Check sheet for the modelled part. Datum: model origin and axes. Units: mm. Face numbers are marked on the shaded views. Round coordinates to 2 decimals unless told otherwise and drop trailing zeros. Write each loop counter-clockwise with the first axis right and the second up, starting at its lowest first coordinate (ties: lowest second). Pieces come first, ordered by that corner, then holes. Notation, with made-up numbers: (-31.75, 80) -> (-19.75, 80) arc R22 cw to (-19.75, 107) -> close; hole circle Ø3 at (-9.5, 43.5). An arc over 180 degrees is marked (long way). One line per item, written item: value.
from build123d import *

# Parameters (mm, degrees)
F1_DEPTH  = 1600
F3_DEPTH  = 1.5
F5_DEPTH  = 13.5
F6_W      = 507
F6_H      = 1.5
F7_ANGLE  = 90
F8_W      = 507
F8_H      = 1.5
F9_DEPTH  = 13.5
F10_W     = 1.5
F10_H     = 28.5
F12_W     = 1.5
F12_H     = 28.5
F15_DEPTH = 1.5
F16_W     = 500
F16_H     = 1.5
F17_DEPTH = 38.5
F18_R     = 5
F19_W     = 30
F19_H     = 30
F20_DEPTH = 865.5
F21_W     = 490
F21_H     = 30
F22_DEPTH = 936.5
F23_W     = 430
F23_H     = 30
F24_DEPTH = 30


with BuildPart() as f1:
    # F0 (on Front) → F1 (new body)
    with BuildSketch(Plane.XZ):
        with BuildLine():
            Line((-285, 28.5), (-285, 0))
            Line((-285, 0), (-283.5, 0))
            Line((-283.5, 0), (-283.5, 28.5))
            Line((-283.5, 28.5), (-256.5, 28.5))
            Line((-256.5, 28.5), (-256.5, 3))
            ThreePointArc((-256.5, 3), (-255.6213203436, 0.8786796564), (-253.5, 0))
            Line((-253.5, 0), (253.5, 0))
            ThreePointArc((253.5, 0), (255.6213203436, 0.8786796564), (256.5, 3))
            Line((256.5, 3), (256.5, 28.5))
            Line((256.5, 28.5), (283.5, 28.5))
            Line((283.5, 28.5), (283.5, 0))
            Line((283.5, 0), (285, 0))
            Line((285, 0), (285, 28.5))
            ThreePointArc((285, 28.5), (284.5606601718, 29.5606601718), (283.5, 30))
            Line((283.5, 30), (256.5, 30))
            ThreePointArc((256.5, 30), (255.4393398282, 29.5606601718), (255, 28.5))
            Line((255, 28.5), (255, 3))
            ThreePointArc((255, 3), (254.5606601718, 1.9393398282), (253.5, 1.5))
            Line((253.5, 1.5), (-253.5, 1.5))
            ThreePointArc((-253.5, 1.5), (-254.5606601718, 1.9393398282), (-255, 3))
            Line((-255, 3), (-255, 28.5))
            ThreePointArc((-255, 28.5), (-255.4393398282, 29.5606601718), (-256.5, 30))
            Line((-256.5, 30), (-283.5, 30))
            ThreePointArc((-283.5, 30), (-284.5606601718, 29.5606601718), (-285, 28.5))
        make_face()
    extrude(amount=F1_DEPTH)

    # F2 (on face) → F3 (join)
    with BuildSketch(Plane(origin=(0, 0, 0), x_dir=(-1, 0, 0), z_dir=(0, 1, 0))):
        with BuildLine():
            ThreePointArc((-283.5, 30), (-284.5606601718, 29.5606601718), (-285, 28.5))
            Line((-285, 28.5), (-285, 0))
            Line((-285, 0), (285, 0))
            Line((285, 0), (285, 28.5))
            ThreePointArc((285, 28.5), (284.5606601718, 29.5606601718), (283.5, 30))
            Line((283.5, 30), (-283.5, 30))
        make_face()
    extrude(amount=F3_DEPTH)

    # F4 (on face) → F5 (join)
    with BuildSketch(Plane.XZ.offset(1600)):
        with BuildLine():
            ThreePointArc((253.5, 0), (255.6213203436, 0.8786796564), (256.5, 3))
            Line((256.5, 3), (256.5, 15))
            Line((256.5, 15), (255, 15))
            Line((255, 15), (255, 3))
            ThreePointArc((255, 3), (254.5606601718, 1.9393398282), (253.5, 1.5))
            Line((253.5, 1.5), (-253.5, 1.5))
            ThreePointArc((-253.5, 1.5), (-254.5606601718, 1.9393398282), (-255, 3))
            Line((-255, 3), (-255, 15))
            Line((-255, 15), (-256.5, 15))
            Line((-256.5, 15), (-256.5, 3))
            ThreePointArc((-256.5, 3), (-255.6213203436, 0.8786796564), (-253.5, 0))
            Line((-253.5, 0), (253.5, 0))
        make_face()
    extrude(amount=F5_DEPTH)

    # F6 (on face) → F7 (revolve)
    with BuildSketch(Plane.XZ.offset(1613.5)):
        with Locations((0, 0.75)):
            Rectangle(F6_W, F6_H)
    revolve(axis=Axis((0, -1613.5, 0), (1, 0, 0)), revolution_arc=F7_ANGLE)

    # F8 (on face) → F9 (join)
    with BuildSketch(Plane(origin=(0, 0, 0), x_dir=(1, 0, 0), z_dir=(0, 0, -1))):
        with Locations((0, 1614.25)):
            Rectangle(F8_W, F8_H)
    extrude(amount=F9_DEPTH)

    # F10 (on face) → F11 (join, up to the next surface of F1)
    with BuildSketch(Plane(origin=(283.5, 0, 0), x_dir=(0, -1, 0), z_dir=(-1, 0, 0))):
        with Locations((1599.25, 14.25)):
            Rectangle(F10_W, F10_H)
    extrude(until=Until.NEXT)

    # F12 (on face) → F13 (join, up to the next surface of F1)
    with BuildSketch(Plane.YZ.offset(-283.5)):
        with Locations((-1599.25, 14.25)):
            Rectangle(F12_W, F12_H)
    extrude(until=Until.NEXT)

    # F14 (on face) → F15 (join)
    with BuildSketch(Plane(origin=(0, 0, 0), x_dir=(1, 0, 0), z_dir=(0, 0, -1))):
        with BuildLine():
            Line((250, 1570.5), (250, 1605.5))
            Line((250, 1605.5), (-250, 1605.5))
            Line((-250, 1605.5), (-250, 1570.5))
            ThreePointArc((-250, 1570.5), (-248.5355339059, 1566.9644660941), (-245, 1565.5))
            Line((-245, 1565.5), (245, 1565.5))
            ThreePointArc((245, 1565.5), (248.5355339059, 1566.9644660941), (250, 1570.5))
        make_face()
    extrude(amount=F15_DEPTH)

    # F16 (on face) → F17 (join)
    with BuildSketch(Plane(origin=(0, 0, -1.5), x_dir=(1, 0, 0), z_dir=(0, 0, -1))):
        with Locations((0, 1604.75)):
            Rectangle(F16_W, F16_H)
    extrude(amount=F17_DEPTH)

    # F18
    f18_edges = [f1.edges().sort_by_distance(p)[0] for p in [
        (-250, -1604.75, -40),
        (250, -1604.75, -40),
    ]]
    fillet(f18_edges, radius=F18_R)

    # F19 (on face) → F20 (join)
    with BuildSketch(Plane(origin=(0, 0, 0), x_dir=(1, 0, 0), z_dir=(0, 0, -1))):
        with Locations((-230, 1525)):
            Rectangle(F19_W, F19_H)
        with Locations((230, 1525)):
            Rectangle(F19_W, F19_H)
    extrude(amount=F20_DEPTH)

    # F21 (on face) → F22 (join)
    with BuildSketch(Plane.XZ.offset(1540)):
        with Locations((0, -730.5)):
            Rectangle(F21_W, F21_H)
    extrude(amount=-F22_DEPTH)

    # F23 (on face) → F24 (join)
    with BuildSketch(Plane(origin=(0, -603.5, 0), x_dir=(-1, 0, 0), z_dir=(0, 1, 0))):
        with Locations((0, -730.5)):
            Rectangle(F23_W, F23_H)
    extrude(amount=F24_DEPTH)


solid = f1.part
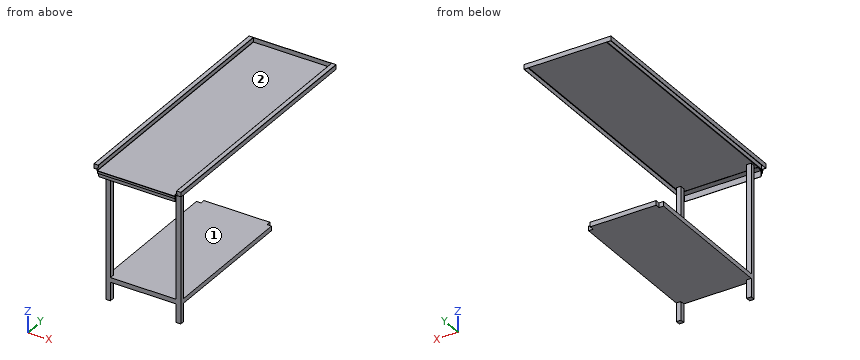
Item 1: Sectioned sample at A-A (y = -1485). Enter the section's corners in (x, z), then the cut area to 3 significant figures.
Result set:
outline: (-285, 0) -> (-283.5, 0) -> (-283.5, 28.5) -> (-256.5, 28.5) -> (-256.5, 3) arc R3 ccw to (-253.5, 0) -> (253.5, 0) arc R3 ccw to (256.5, 3) -> (256.5, 28.5) -> (283.5, 28.5) -> (283.5, 0) -> (285, 0) -> (285, 28.5) arc R1.5 ccw to (283.5, 30) -> (256.5, 30) arc R1.5 ccw to (255, 28.5) -> (255, 3) arc R1.5 cw to (253.5, 1.5) -> (-253.5, 1.5) arc R1.5 cw to (-255, 3) -> (-255, 28.5) arc R1.5 ccw to (-256.5, 30) -> (-283.5, 30) arc R1.5 ccw to (-285, 28.5) -> close; (-245, -745.5) -> (245, -745.5) -> (245, -715.5) -> (-245, -715.5) -> close
area: 15,700 mm^2
Item 2: Sectioned sample at D-D (y = -449.5). Enter the section's corners in (x, z), then the cut area to 3 significant figures.
Result set:
outline: (-285, 0) -> (-283.5, 0) -> (-283.5, 28.5) -> (-256.5, 28.5) -> (-256.5, 3) arc R3 ccw to (-253.5, 0) -> (253.5, 0) arc R3 ccw to (256.5, 3) -> (256.5, 28.5) -> (283.5, 28.5) -> (283.5, 0) -> (285, 0) -> (285, 28.5) arc R1.5 ccw to (283.5, 30) -> (256.5, 30) arc R1.5 ccw to (255, 28.5) -> (255, 3) arc R1.5 cw to (253.5, 1.5) -> (-253.5, 1.5) arc R1.5 cw to (-255, 3) -> (-255, 28.5) arc R1.5 ccw to (-256.5, 30) -> (-283.5, 30) arc R1.5 ccw to (-285, 28.5) -> close
area: 1,020 mm^2
Item 3: Release check for a two-part mould opening along Z. For the marked faces 1 and 2 record: pulls with the +Z half, pulls with the -Z half, needs draft (parallel to the pull), parting line crosses it, or undercut.
Result set:
face 1: undercut
face 2: pulls with the +Z half
Item 4: Sectioned sample at B-B (x = -104). Enter the section's corners in (y, z), then the cut area to 3 significant figures.
Result set:
outline: (-1615, -13.5) -> (-1613.5, -13.5) -> (-1613.5, 0) -> (-1605.5, 0) -> (-1605.5, -40) -> (-1604, -40) -> (-1604, -1.5) -> (-1565.5, -1.5) -> (-1565.5, 0) -> (1.5, 0) -> (1.5, 30) -> (0, 30) -> (0, 1.5) -> (-1613.5, 1.5) arc R1.5 ccw to (-1615, 0) -> close; (-1540, -745.5) -> (-573.5, -745.5) -> (-573.5, -715.5) -> (-1540, -715.5) -> close
area: 31,600 mm^2
Item 5: Sectioned sample at C-C (z = -572). Enter the section's corners in (x, y), then the cut area to 3 significant figures.
Result set:
outline: (-245, -1540) -> (-215, -1540) -> (-215, -1510) -> (-245, -1510) -> close; (215, -1540) -> (245, -1540) -> (245, -1510) -> (215, -1510) -> close
area: 1,800 mm^2
Item 6: Material ranges on line 1 along Z through (x, y) = (-42.5, -904.5); line 2 along Y through (x, z) = (232, -784); line 3 along Z through (x, y) = (-169.5, -477), recorded low to high.
Result set:
line 1: -745.5 to -715.5, 0 to 1.5
line 2: -1540 to -1510
line 3: 0 to 1.5
Item 7: Depth check by flat-ended pin: pin 1 (6 mm diameter, centred on x = 105, y = -1212, fed in from -Z); pin 2 (19 mm diameter, centred on x = -116, y = -1591, fed in from -Z); pin 3 (15 mm diameter, centred on y = -594, z = -738, fed in from +X). Enter the tip coordinate at first touch or a pass-through.
Result set:
pin 1: z = -745.5
pin 2: z = -1.5
pin 3: x = 215
